from build123d import *

# Parameters (mm, degrees)
EXTRUDE_6_DEPTH      = 33
CUT_EXTRUDE_START    = 3
CUT_EXTRUDE_2_DEPTH  = 27
EXTRUDE_START        = 6.5
SKETCH_7_W           = 32
SKETCH_7_H           = 13
EXTRUDE_7_DEPTH      = 20
EXTRUDE_START_2      = 1.5
SKETCH_11_W          = 13
SKETCH_11_H          = 2.5
EXTRUDE_15_DEPTH     = 30
CUT_EXTRUDE_START_2  = 180
CUT_EXTRUDE_3_DEPTH  = 10
SKETCH_13_R          = 1.5
CUT_EXTRUDE_4_DEPTH  = 30
SKETCH_14_W          = 15
SKETCH_14_H          = 2
CUT_EXTRUDE_5_DEPTH  = 30
EXTRUDE_START_3      = 11.5
SKETCH_15_W          = 67.299618531
SKETCH_15_H          = 10
EXTRUDE_16_DEPTH     = 10
CUT_EXTRUDE_START_3  = 17
CUT_EXTRUDE_7_DEPTH  = 75
CUT_EXTRUDE_START_4  = 13
CUT_EXTRUDE_9_DEPTH  = 5
SKETCH_20_W          = 16.6
SKETCH_20_H          = 24.7
CUT_EXTRUDE_10_DEPTH = 5
SKETCH_21_R          = 6
CUT_EXTRUDE_11_DEPTH = 5
SKETCH_22_W          = 51
SKETCH_22_H          = 47
CUT_EXTRUDE_12_DEPTH = 27


with BuildPart() as part:
    # Sketch 1 → Extrude 6 (new body)
    with BuildSketch(Plane.XY):
        with BuildLine():
            Line((4.299618531, 175.402841826), (4.299618531, 188.402841826))
            Line((4.299618531, 188.402841826), (65.299618531, 188.402841826))
            Line((65.299618531, 188.402841826), (86.299618531, 168.402841826))
            Line((86.299618531, 168.402841826), (86.299619, 0))
            Line((86.299619, 0), (86.299619, -28))
            Line((86.299619, -28), (0, -28))
            Line((0, -28), (0, 0))
            ThreePointArc((0, 0), (37.229295141, 21.561020186), (55.173142182, 60.662380285))
            ThreePointArc((55.173142182, 60.662380285), (56.797307883, 87.162380285), (55.173142182, 113.662380285))
            ThreePointArc((55.173142182, 113.662380285), (38.726552267, 151.940422917), (4.299618531, 175.402841826))
        make_face()
    extrude(amount=EXTRUDE_6_DEPTH)

    # Sketch 5 → Cut-Extrude 2 (cut)
    with BuildSketch(Plane.XY.offset(CUT_EXTRUDE_START)):
        Polygon((24.099618531, 175.402841826), (4.299618531, 175.402841826), (4.299618531, 169.136823089), (-18.700381469, 169.136823089), (-18.700381469, -23.02337805), (14, -23.02337805), (14, 8.47662195), (81.178938205, 8.47662195), (81.178938205, 169.136823089), (64.099618531, 185.402841826), (24.099618531, 185.402841826), align=None)
    extrude(amount=CUT_EXTRUDE_2_DEPTH, mode=Mode.SUBTRACT)

    # Sketch 7 → Extrude 7 (add)
    with BuildSketch(Plane.XY.offset(EXTRUDE_START)):
        with Locations((-11.700381469, 181.902841826)):
            Rectangle(SKETCH_7_W, SKETCH_7_H)
    extrude(amount=EXTRUDE_7_DEPTH)

    # Sketch 11 → Extrude 15 (add)
    with BuildSketch(Plane.XY.offset(EXTRUDE_START_2)):
        with Locations((3.799618531, 174.152841826)):
            Rectangle(SKETCH_11_W, SKETCH_11_H)
    extrude(amount=EXTRUDE_15_DEPTH)

    # Sketch 12 → Cut-Extrude 3 (cut)
    with BuildSketch(Plane(origin=(0, 0, 0), x_dir=(1, 0, 0), z_dir=(0, 1, 0)).offset(CUT_EXTRUDE_START_2)):
        with BuildLine():
            Line((1.142696527, -30.654700538), (1.642696527, -30.366025404))
            ThreePointArc((1.642696527, -30.366025404), (1.142696527, -28.5), (0.642696527, -30.366025404))
            Line((0.642696527, -30.366025404), (1.142696527, -30.654700538))
        make_face()
        with BuildLine():
            Line((1.142696527, -4.654700538), (1.642696527, -4.366025404))
            ThreePointArc((1.642696527, -4.366025404), (1.142696527, -2.5), (0.642696527, -4.366025404))
            Line((0.642696527, -4.366025404), (1.142696527, -4.654700538))
        make_face()
    extrude(amount=-CUT_EXTRUDE_3_DEPTH, mode=Mode.SUBTRACT)

    # Sketch 13 → Cut-Extrude 4 (cut)
    with BuildSketch(Plane.XY):
        with Locations((-2.700381469, 183.402841826)):
            Circle(SKETCH_13_R)
    extrude(amount=CUT_EXTRUDE_4_DEPTH, mode=Mode.SUBTRACT)

    # Sketch 14 → Cut-Extrude 5 (cut)
    with BuildSketch(Plane.XY):
        with Locations((-20.200381469, 187.402841826)):
            Rectangle(SKETCH_14_W, SKETCH_14_H)
    extrude(amount=CUT_EXTRUDE_5_DEPTH, mode=Mode.SUBTRACT)

    # Sketch 15 → Extrude 16 (add)
    with BuildSketch(Plane.XY.offset(EXTRUDE_START_3)):
        with Locations((47.649809735, 1.5)):
            Rectangle(SKETCH_15_W, SKETCH_15_H)
    extrude(amount=EXTRUDE_16_DEPTH)

    # Sketch 17 → Cut-Extrude 7 (cut)
    with BuildSketch(Plane(origin=(0, 0, 0), x_dir=(0, 0, -1), z_dir=(1, 0, 0)).offset(CUT_EXTRUDE_START_3)):
        with BuildLine():
            Line((-21.118802154, 1.5), (-19.964101615, 3.5))
            ThreePointArc((-19.964101615, 3.5), (-12.5, 1.5), (-19.964101615, -0.5))
            Line((-19.964101615, -0.5), (-21.118802154, 1.5))
        make_face()
    extrude(amount=CUT_EXTRUDE_7_DEPTH, mode=Mode.SUBTRACT)

    # Sketch 18 → Cut-Extrude 9 (cut)
    with BuildSketch(Plane(origin=(0, 0, 0), x_dir=(0, 0, -1), z_dir=(1, 0, 0)).offset(CUT_EXTRUDE_START_4)):
        with BuildLine():
            Line((-18.809401077, 1.5), (-18.232050808, 2.5))
            ThreePointArc((-18.232050808, 2.5), (-14.5, 1.5), (-18.232050808, 0.5))
            Line((-18.232050808, 0.5), (-18.809401077, 1.5))
        make_face()
    extrude(amount=CUT_EXTRUDE_9_DEPTH, mode=Mode.SUBTRACT)

    # Sketch 20 → Cut-Extrude 10 (cut)
    with BuildSketch(Plane(origin=(0, 188.402841826, 0), x_dir=(1, 0, 0), z_dir=(0, 1, 0))):
        with Locations((40.95, -16.5)):
            Rectangle(SKETCH_20_W, SKETCH_20_H)
        with BuildLine():
            Line((30, -29.143375673), (30.625, -28.782531755))
            ThreePointArc((30.625, -28.782531755), (30, -26.45), (29.375, -28.782531755))
            Line((29.375, -28.782531755), (30, -29.143375673))
        make_face()
        with BuildLine():
            Line((30, -6.743375673), (30.625, -6.382531755))
            ThreePointArc((30.625, -6.382531755), (30, -4.05), (29.375, -6.382531755))
            Line((29.375, -6.382531755), (30, -6.743375673))
        make_face()
        with BuildLine():
            Line((51.9, -6.743375673), (52.525, -6.382531755))
            ThreePointArc((52.525, -6.382531755), (51.9, -4.05), (51.275, -6.382531755))
            Line((51.275, -6.382531755), (51.9, -6.743375673))
        make_face()
        with BuildLine():
            Line((51.9, -29.143375673), (52.525, -28.782531755))
            ThreePointArc((52.525, -28.782531755), (51.9, -26.45), (51.275, -28.782531755))
            Line((51.275, -28.782531755), (51.9, -29.143375673))
        make_face()
    extrude(amount=-CUT_EXTRUDE_10_DEPTH, mode=Mode.SUBTRACT)

    # Sketch 21 → Cut-Extrude 11 (cut)
    with BuildSketch(Plane(origin=(125.147492247, 131.404866859, 0), x_dir=(0, 0, -1), z_dir=(0.689655172, 0.724137931, 0))):
        with Locations((-16.5, 68.147063703)):
            Circle(SKETCH_21_R)
    extrude(amount=-CUT_EXTRUDE_11_DEPTH, mode=Mode.SUBTRACT)

    # Sketch 22 → Cut-Extrude 12 (cut)
    with BuildSketch(Plane.XY.offset(CUT_EXTRUDE_START)):
        with Locations((55.799619, -1.5)):
            Rectangle(SKETCH_22_W, SKETCH_22_H)
    extrude(amount=CUT_EXTRUDE_12_DEPTH, mode=Mode.SUBTRACT)


solid = part.part
Could you check a few things on this model? Use its own coordinates, in mm. A direction names the side the tool comes from. Round coordinates to 2 decimals unless told otherwise and drop trailing zeros. Loops run counter-clockwise (first coordinate to the right, second up) from the corner with the lowest first, then second, coordinate; pieces in that order, holes last. Notation, with made-up numbers: (74.5, 51) - (122.5, 51) arc R19 cw to (122.5, 79) - close; hole circle Ø2 at (21, 85.5). An arc over 180 degrees is marked (long way). Write item = value, one per line.
1) Imagine slicing it at C-C (x = 8). Please give me the cut outline in (y, z), and give its area (3 significant figures).
Computed:
outline = (-28, 0) - (2.26, 0) - (2.26, 3) - (-23.02, 3) - (-23.02, 30) - (2.26, 30) - (2.26, 33) - (-28, 33) - close; (172.9, 1.5) - (174.09, 1.5) - (174.09, 0) - (188.4, 0) - (188.4, 33) - (174.09, 33) - (174.09, 31.5) - (172.9, 31.5) - close
area = 824 mm2
2) I need wall thicknesses on line 1 along Z through (x, y) = (30, 187.6); line 2 along X through (y, z) = (1.5, 9.5); line 3 along Z through (x, y) = (51, 187). Which ranges of each line are inside material? Lowest first, please. Write a range as from..to.
Computed:
line_1 = 0..4.05, 6.74..26.45, 29.14..33
line_2 = 14..30.3, 81.3..86.3
line_3 = 0..4.43, 6.17..26.83, 28.57..33
3) On a 3-axis mill with a long thin cutter (end or side, diameter ignored), from which of +Z, -Z, +X, -X, +Y, -Y can I reach the whole of each face in a straight line? I mean faces 5 (the flat face through (4, 172.903, 16)), 6 (the flat face through (61, 82, 3)), 7 (the flat face through (17, 3.3, 17.7)), 8 (the flat face through (4.3, 182, 30)), 9 (the flat face through (7, -9, 3)). Say none if no direction works.
Computed:
face_5 = +Z, -Z, -X
face_6 = none
face_7 = +X
face_8 = +Z, -X, +Y
face_9 = -X
4) If we mould it in two halves opening along Y, with no side actions, what happens to faces 1 (the cylindrical face through (39.101, 151.483, 31.479)), 2 (the flat face through (4.3, 182, 3)), 3 (the flat face through (1, 175.403, 5)), 4 (the cylindrical face through (23.6, 1.6, 12.5))? For each: pulls with the +Y half, pulls with the -Y half, needs draft (parallel to the pull), parting line crosses it, or undercut.
Computed:
face_1 = undercut
face_2 = needs draft
face_3 = pulls with the +Y half
face_4 = undercut
5) Imagine slicing it at D-D (x = -15.5). Please give me the cut outline in (y, z), and give its area (3 significant figures).
Computed:
outline = (175.4, 6.5) - (186.4, 6.5) - (186.4, 26.5) - (175.4, 26.5) - close
area = 220 mm2
6) I'm going to push flat-ended pins straight in: P1, Ø4, axis at y = 53.5, z = 5.5, coming from the -X side; P2, Ø6, axis at y = 80.5, z = 28, coming from the -X side; P3, Ø2.5, axis at y = 186.5, z = 21, coming from the +X side. Where does each tip first touch, or does it pass through?
Computed:
P1 = 81.18
P2 = 56.61
P3 = 68.61
7) Imagine slicing it at A-A (x = 37). Please give me the cut outline in (y, z).
Computed:
outline = (-28, 0) - (21.31, 0) - (21.31, 3) - (-25, 3) - (-25, 30) - (21.31, 30) - (21.31, 33) - (-28, 33) - close; (153.96, 0) - (188.4, 0) - (188.4, 4.15) - (185.4, 4.15) - (185.4, 3) - (153.96, 3) - close; (153.96, 30) - (185.4, 30) - (185.4, 28.85) - (188.4, 28.85) - (188.4, 33) - (153.96, 33) - close
8) Imagine slicing it at B-B (y = 139). Please give me the cut outline in (x, z), and give its area (3 significant figures).
Computed:
outline = (47.29, 0) - (86.3, 0) - (86.3, 33) - (47.29, 33) - (47.29, 30) - (81.18, 30) - (81.18, 3) - (47.29, 3) - close
area = 372 mm2
